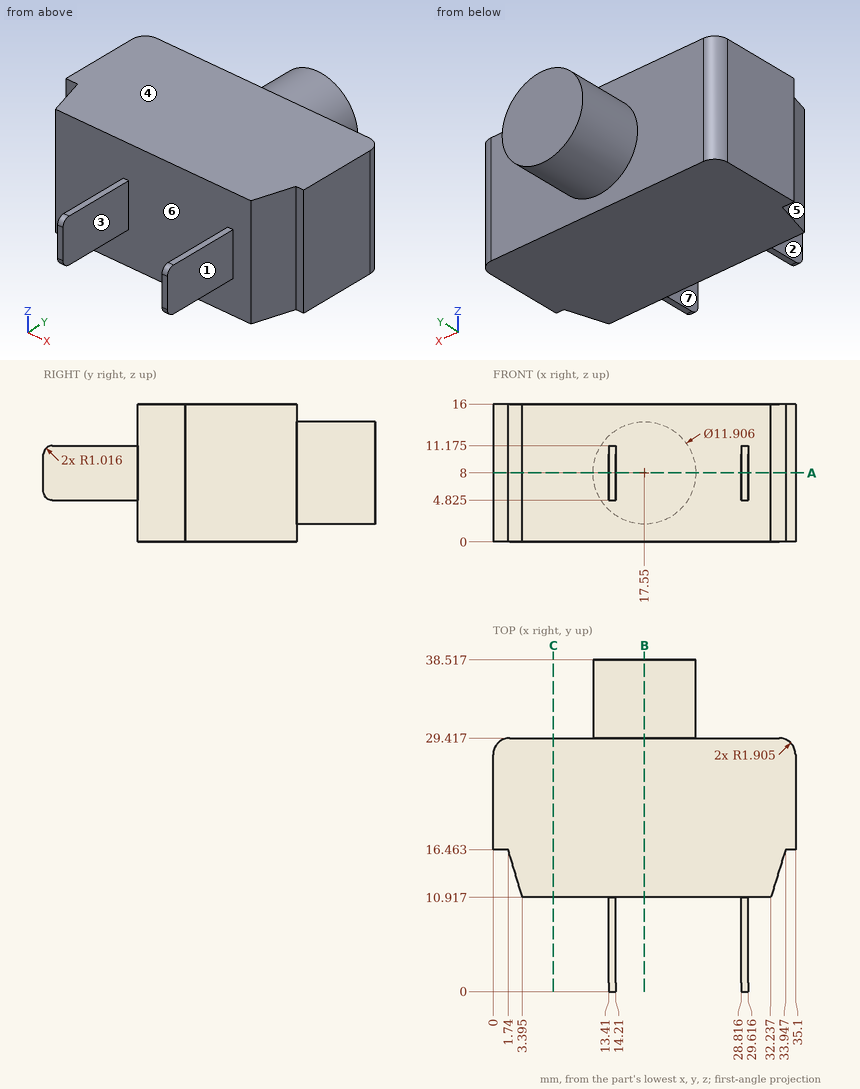
Geometry check sheet. Reference: drawing and pictorial views, mm from the part's lowest x, y, z. A direction names the side the tool comes from. Give positions to 0.01 mm unless a question says otherwise; leave off trailing zeros. Order: outer loops, then holes, each group sorted by start corner. A loop starts at its lowest first (then second) coordinate and runs counter-clockwise, first axis right, second up. Notation, with made-up numbers: M 36.25,43 L 75.25,43 A36 cw 75.25,79 Z; hole C 72.25,-5.5 d4. An arc over 180 degrees is marked long. Use one line per item in the form item = value. Start each with the question number.
Q1. Section check C-C (x = 7). Enter the section's corners in (y, z), then the cut area to 3 significant figures.
Q2. Access from +Z, -Z, +X, -X, +Y, -Y to the whole of each face (thin tool, end or side, straight path). Record for the marked faces 1, 2 and 3.
Q3. Go/stop test with flat-tipped pins: pin 1 Ø3 at (y, z) = (14.5, 3) entering from +X (1 decimal); pin 2 Ø1 at (x, z) = (24.5, 3.5) entering from +Y; pin 3 Ø7 at (y, z) = (6.5, 9) entering from +X; pin 4 Ø2 at (x, y) = (31.5, 29) entering from -Z. Record where each tip stops, or that it passes through.
Q4. Section check A-A (z = 8). Enter the section's corners in (x, y) (1 decimal), then the cut area to 3 significant figures.
Q5. Scan lines: line 1 along X through (y, z) = (5, 9) (1 decimal); line 2 along Y through (x, z) = (4.5, 13.5); line 3 along Y through (x, z) = (29, 8). Record each from-to range of solid material in increasing order. Write a range as [from, to].
Q6. Section check B-B (x = 17.55). Enter the section's corners in (y, z), then the cut area to 3 significant figures.
Q7. Mould release check, pull along X, two halves, no side actions. Record for the marked faces 4, 5, 6 and 7: +X half, -X half, draft (parallel to the pull), parting line (faces both ways), or undercut.
Evaluation:
q1.outline = M 10.92,0 L 29.42,0 L 29.42,16 L 10.92,16 Z
q1.area = 296 mm2
q2.face_1 = +Z, -Z, +X, -Y
q2.face_2 = +Z, -Z, -X, -Y
q2.face_3 = +Z, -Z, -Y
q3.pin_1 = 33.8
q3.pin_2 = 29.42
q3.pin_3 = 29.62
q3.pin_4 = 0
q4.outline = M 0,16.5 L 1.7,16.5 L 3.4,10.9 L 13.4,10.9 L 13.4,0 L 14.2,0 L 14.2,10.9 L 28.8,10.9 L 28.8,0 L 29.6,0 L 29.6,10.9 L 32.2,10.9 L 33.9,16.5 L 35.1,16.5 L 35.1,27.5 A1.9 ccw 33.2,29.4 L 23.5,29.4 L 23.5,38.5 L 11.6,38.5 L 11.6,29.4 L 1.9,29.4 A1.9 ccw 0,27.5 Z
q4.area = 748 mm2
q5.line_1 = [13.4, 14.2], [28.8, 29.6]
q5.line_2 = [10.92, 29.42]
q5.line_3 = [0, 29.42]
q6.outline = M 10.92,0 L 29.42,0 L 29.42,2.05 L 38.52,2.05 L 38.52,13.95 L 29.42,13.95 L 29.42,16 L 10.92,16 Z
q6.area = 404 mm2
q7.face_4 = draft
q7.face_5 = -X half
q7.face_6 = undercut
q7.face_7 = undercut
